Input: part model. Units: mm. Frame: model coordinates. Face numbers are marked on the shaded views. A direction names the side the tool comes from. Round coordinates to 2 decimals unless told otherwise and drop trailing zeros. Loops run counter-clockwise (first coordinate to the right, second up) from the corner with the lowest first, then second, coordinate; pieces in that order, holes last. Notation, with made-up numbers: M 1.5,56.25 L 57.5,56.25 A16 ccw 57.5,66.25 Z; hole C -2.5,19 d6. An arc over 180 degrees is marked long. Return JSON: item names as keys, results as strings. Group by question number.
1) Contact query for flat-ended pins moving along their axis: P1, Ø6.5, axis at x = -15.5, z = -2.5, coming from the +Y side; P2, Ø4.5, axis at x = 34, y = 34, coming from the +Z side; P3, Ø4, axis at x = 35, y = -36, coming from the +Z side. Output: stop coordinate, or through.
2) Section B-B (y = 0). Output: boundary loops of the cut face in (x, z).
3) Material intervals for line 1 (X direction, y = -32.5, z = 16.25) (3 decimals); line 2 (Y direction, x = 32, z = 8); line 3 (X direction, y = -25.5, z = 4.5), sorted ascending. Write a range as from..to.
4) Mould query, pull axis X, two halves, no side actions, for the marked faces 4, 5 and 6. Classes: +X half, -X half, draft (parallel to the pull), parting line (faces both ways), or undercut.
5) Section D-D (z = 7). Output: boundary loops of the cut face in (x, y), plus the area to 3 significant figures.
6) Section A-A (x = 0). Output: boundary loops of the cut face in (y, z), plus the area to 3 significant figures.
7) Access query for the marked faces 1, 2 and 3. Directions: +Z, -Z, +X, -X, +Y, -Y. A direction counts if a zero-diameter tool reaches every point of the face in a straight line with its end or side. Return the directions, or none.
8) Section C-C (z = 16.5). Output: boundary loops of the cut face in (x, y), plus the area to 3 significant figures.
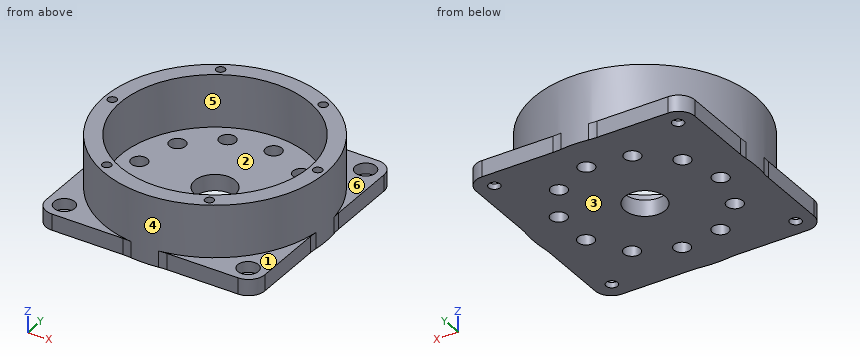
from build123d import *

# Parameters (mm, degrees)
SKETCH1_R                                    = 41
SKETCH1_R_2                                  = 3
BOSS_EXTRUDE1_DEPTH                          = 6
BOSS_EXTRUDE2_START                          = 19.4
SKETCH3_R                                    = 41
SKETCH3_R_2                                  = 35
BOSS_EXTRUDE2_DEPTH                          = 19.4
SKETCH5_R                                    = 7.5
CUT_EXTRUDE1_DEPTH                           = 62.142129502
SKETCH6_R                                    = 1.65
CUT_EXTRUDE2_DEPTH                           = 10
BOSS_EXTRUDE3_START                          = -6
SKETCH7_R                                    = 2.1
BOSS_EXTRUDE3_DEPTH                          = 6
FILLET1_R                                    = 6
FILLET2_R                                    = 24
CBORE_FOR_M4_HEX_HEAD_CAP_SCREW1_D           = 4.2
CBORE_FOR_M4_HEX_HEAD_CAP_SCREW1_CBORE_D     = 7.6
CBORE_FOR_M4_HEX_HEAD_CAP_SCREW1_CBORE_DEPTH = 4
CIRPATTERN1_COUNT                            = 4
FILLET1_OF_CIRPATTERN1_R                     = 6
FILLET2_OF_CIRPATTERN1_R                     = 24


with BuildPart() as part:
    # Sketch1 → Boss-Extrude1 (new body)
    with BuildSketch(Plane(origin=(0, 0, 0), x_dir=(0, 1, 0), z_dir=(0, 0, 1))):
        with Locations(Location((0, 0, 0), (0, 0, 270))):
            Circle(SKETCH1_R)
        with Locations(Location((0, 28, 0), (0, 0, 270))):
            Circle(SKETCH1_R_2, mode=Mode.SUBTRACT)
        with Locations(Location((15.137942889, 23.555098919, 0), (0, 0, 270))):
            Circle(SKETCH1_R_2, mode=Mode.SUBTRACT)
        with Locations(Location((25.46969587, 11.631620364, 0), (0, 0, 270))):
            Circle(SKETCH1_R_2, mode=Mode.SUBTRACT)
        with Locations(Location((27.715000373, -3.984815472, 0), (0, 0, 270))):
            Circle(SKETCH1_R_2, mode=Mode.SUBTRACT)
        with Locations(Location((21.160988082, -18.33610055, 0), (0, 0, 270))):
            Circle(SKETCH1_R_2, mode=Mode.SUBTRACT)
        with Locations(Location((7.888511592, -26.865803261, 0), (0, 0, 270))):
            Circle(SKETCH1_R_2, mode=Mode.SUBTRACT)
        with Locations(Location((-7.888511592, -26.865803261, 0), (0, 0, 270))):
            Circle(SKETCH1_R_2, mode=Mode.SUBTRACT)
        with Locations(Location((-21.160988082, -18.33610055, 0), (0, 0, 270))):
            Circle(SKETCH1_R_2, mode=Mode.SUBTRACT)
        with Locations(Location((-27.715000373, -3.984815472, 0), (0, 0, 270))):
            Circle(SKETCH1_R_2, mode=Mode.SUBTRACT)
        with Locations(Location((-25.46969587, 11.631620364, 0), (0, 0, 270))):
            Circle(SKETCH1_R_2, mode=Mode.SUBTRACT)
        with Locations(Location((-15.137942889, 23.555098919, 0), (0, 0, 270))):
            Circle(SKETCH1_R_2, mode=Mode.SUBTRACT)
    extrude(amount=-BOSS_EXTRUDE1_DEPTH)

    # Sketch3 → Boss-Extrude2 (add)
    with BuildSketch(Plane.XY.offset(BOSS_EXTRUDE2_START)):
        Circle(SKETCH3_R)
        Circle(SKETCH3_R_2, mode=Mode.SUBTRACT)
    extrude(amount=-BOSS_EXTRUDE2_DEPTH)

    # Sketch5 → Cut-Extrude1 (cut, through all)
    with BuildSketch(Plane.XY):
        Circle(SKETCH5_R)
    extrude(amount=-CUT_EXTRUDE1_DEPTH, mode=Mode.SUBTRACT)

    # Sketch6 → Cut-Extrude2 (cut)
    with BuildSketch(Plane.XY.offset(19.4)):
        with Locations((-38, 0)):
            Circle(SKETCH6_R)
        with Locations((-19, 32.908965344)):
            Circle(SKETCH6_R)
        with Locations((19, 32.908965344)):
            Circle(SKETCH6_R)
        with Locations((38, 0)):
            Circle(SKETCH6_R)
        with Locations((19, -32.908965344)):
            Circle(SKETCH6_R)
        with Locations((-19, -32.908965344)):
            Circle(SKETCH6_R)
    extrude(amount=-CUT_EXTRUDE2_DEPTH, mode=Mode.SUBTRACT)

    # Sketch7 → Boss-Extrude3 (add)
    with BuildSketch(Plane(origin=(0, 0, -6), x_dir=(1, 0, 0), z_dir=(0, 0, -1)).offset(BOSS_EXTRUDE3_START)):
        with BuildLine():
            Line((40.484037132, 40.484037132), (6.484037132, 40.484037132))
            ThreePointArc((6.484037132, 40.484037132), (28.991378029, 28.991378029), (40.484037132, 6.484037132))
            Line((40.484037132, 6.484037132), (40.484037132, 40.484037132))
        make_face()
        with Locations(Location((34, 34, 0), (0, 0, 180))):
            Circle(SKETCH7_R, mode=Mode.SUBTRACT)
    boss_extrude3 = extrude(amount=BOSS_EXTRUDE3_DEPTH)

    # Fillet1
    fillet1_edges = [part.edges().sort_by_distance(p)[0] for p in [
        (40.484037132, -40.484037132, -3),
    ]]
    fillet(fillet1_edges, radius=FILLET1_R)

    # Fillet2
    fillet2_edges = [part.edges().sort_by_distance(p)[0] for p in [
        (6.484037132, -40.484037132, -3),
        (40.484037132, -6.484037132, -3),
    ]]
    fillet(fillet2_edges, radius=FILLET2_R)

    # CBORE for M4 Hex Head Cap Screw1 (through all)
    with Locations(Plane.XY):
        with Locations((34, -34)):
            cbore_for_m4_hex_head_cap_screw1 = CounterBoreHole(CBORE_FOR_M4_HEX_HEAD_CAP_SCREW1_D / 2, CBORE_FOR_M4_HEX_HEAD_CAP_SCREW1_CBORE_D / 2, CBORE_FOR_M4_HEX_HEAD_CAP_SCREW1_CBORE_DEPTH)

    # CirPattern1: Boss-Extrude3, CBORE for M4 Hex Head Cap Screw1 ×4 about axis
    cirpattern1_axis = Axis((0, 0, 0), (0, 0, 1))
    add([boss_extrude3.rotate(cirpattern1_axis, i * 360 / CIRPATTERN1_COUNT) for i in range(1, CIRPATTERN1_COUNT)])
    add([cbore_for_m4_hex_head_cap_screw1.rotate(cirpattern1_axis, i * 360 / CIRPATTERN1_COUNT) for i in range(1, CIRPATTERN1_COUNT)], mode=Mode.SUBTRACT)

    # Fillet1 of CirPattern1
    fillet1_of_cirpattern1_edges = [part.edges().sort_by_distance(p)[0] for p in [
        (40.484037132, 40.484037132, -3),
        (-40.484037132, 40.484037132, -3),
        (-40.484037132, -40.484037132, -3),
    ]]
    fillet(fillet1_of_cirpattern1_edges, radius=FILLET1_OF_CIRPATTERN1_R)

    # Fillet2 of CirPattern1
    fillet2_of_cirpattern1_edges = [part.edges().sort_by_distance(p)[0] for p in [
        (40.484037132, 6.484037132, -3),
        (6.484037132, 40.484037132, -3),
        (-6.484037132, 40.484037132, -3),
        (-40.484037132, 6.484037132, -3),
        (-40.484037132, -6.484037132, -3),
        (-6.484037132, -40.484037132, -3),
    ]]
    fillet(fillet2_of_cirpattern1_edges, radius=FILLET2_OF_CIRPATTERN1_R)


solid = part.part
Returned:
{
 "1": {"P1": "stops at y = 40.48", "P2": "stops at z = -4", "P3": "stops at z = 0"},
 "2": {"outline": "M -41,-6 L -31,-6 L -31,0 L -35,0 L -35,19.4 L -36.35,19.4 L -36.35,9.4 L -39.65,9.4 L -39.65,19.4 L -41,19.4 Z; M -25,-6 L -7.5,-6 L -7.5,0 L -25,0 Z; M 7.5,-6 L 41,-6 L 41,19.4 L 39.65,19.4 L 39.65,9.4 L 36.35,9.4 L 36.35,19.4 L 35,19.4 L 35,0 L 7.5,0 Z"},
 "3": {"line 1": "x = -24.995..-20.599, -17.401..-12.99, 12.99..17.401, 20.599..24.995", "line 2": "y = -25.63..-14.18, 14.18..25.63", "line 3": "x = -32.11..-23.97, 23.97..32.11"},
 "4": {"face 4": "parting line", "face 5": "undercut", "face 6": "draft"},
 "5": {"outline": "C 0,0 d82; hole C 0,0 d70", "area": "1,430 mm^2"},
 "6": {"outline": "M -41,-6 L -7.5,-6 L -7.5,0 L -35,0 L -35,19.4 L -41,19.4 Z; M 7.5,-6 L 41,-6 L 41,19.4 L 35,19.4 L 35,0 L 7.5,0 Z", "area": "635 mm^2"},
 "7": {"face 1": "+Z, +X, -Y", "face 2": "+Z", "face 3": "-Z, +X, -X, +Y, -Y"},
 "8": {"outline": "C 0,0 d82; hole C -38,0 d3.3; hole C 0,0 d70; hole C -19,-32.91 d3.3; hole C -19,32.91 d3.3; hole C 19,-32.91 d3.3; hole C 19,32.91 d3.3; hole C 38,0 d3.3", "area": "1,380 mm^2"}
}
